Input: part model. Units: mm. Frame: model coordinates. Face numbers are marked on the shaded views. A direction names the side the tool comes from. Give positions to 0.01 mm unless a question says otherwise; leave off trailing zeros. Loops run counter-clockwise (first coordinate to the right, second up) from the corner with the lowest first, then second, coordinate; pieces in that order, holes last. Notation, with made-up numbers: (19.5, -20.5) - (38.5, -20.5) arc R19 cw to (38.5, -13.5) - close; hole circle Ø8 at (-40, -33). An arc over 180 degrees is marked (long way). Answer as a JSON object with one key per item and string values.
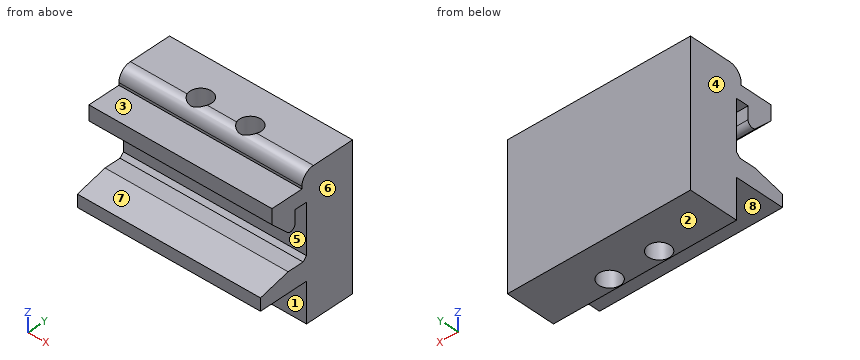
from build123d import *

# Parameters (mm, degrees)
BOSS_EXTRUDE1_DEPTH     = 37
SKETCH3_R               = 2.175
CUT_EXTRUDE1_DEPTH      = 9
CUT_EXTRUDE1_DEPTH_BACK = 21.75


with BuildPart() as part:
    # Sketch2 → Boss-Extrude1 (new body)
    with BuildSketch(Plane(origin=(0, 0, 0), x_dir=(0, 0, -1), z_dir=(1, 0, 0))):
        with BuildLine():
            Line((0, 0), (17.75, 0))
            Line((17.75, 0), (25.75, 0))
            Line((25.75, 0), (25.75, -10))
            Line((25.75, -10), (17.75, -10))
            Line((17.75, -10), (17.75, -20))
            Line((17.75, -20), (15.25, -20))
            Line((15.25, -20), (13.75, -14))
            Line((13.75, -14), (13.75, -10.75))
            Line((13.75, -10.75), (13, -10))
            Line((13, -10), (3, -10))
            Line((3, -10), (3, -12.5))
            Line((3, -12.5), (5.585786438, -12.5))
            ThreePointArc((5.585786438, -12.5), (6.50966597, -13.117316568), (6.292893219, -14.207106781))
            Line((6.292893219, -14.207106781), (3, -17.5))
            Line((3, -17.5), (0, -17.5))
            Line((0, -17.5), (0, -11))
            Line((0, -11), (-0.5, -11))
            ThreePointArc((-0.5, -11), (-2.267766953, -10.267766953), (-3, -8.5))
            Line((-3, -8.5), (-3, 0))
            Line((-3, 0), (0, 0))
        make_face()
    extrude(amount=BOSS_EXTRUDE1_DEPTH)

    # Sketch3 → Cut-Extrude1 (cut, two sides)
    with BuildSketch(Plane(origin=(0, 0, -17.75), x_dir=(-1, 0, 0), z_dir=(0, 0, -1))) as cut_extrude1_sk:
        with Locations((-23.5, -7.7)):
            Circle(SKETCH3_R)
        with Locations((-13.5, -7.7)):
            Circle(SKETCH3_R)
    extrude(amount=CUT_EXTRUDE1_DEPTH, mode=Mode.SUBTRACT)
    extrude(cut_extrude1_sk.sketch, amount=-CUT_EXTRUDE1_DEPTH_BACK, mode=Mode.SUBTRACT)


solid = part.part
Item 1: Material intervals for line 1 (X direction, y = -7.7, z = -12) (3 decimals); line 2 (Z direction, x = 26, y = -11.75); line 3 (X direction, y = -9.25, z = -15.25), sorted ascending. Write a range as [from, to].
Geometry check:
{"line 1": "x = [0, 11.325], [15.675, 21.325], [25.675, 37]", "line 2": "z = [-17.75, -13.75], [-3, 0]", "line 3": "x = [0, 11.97], [15.03, 21.97], [25.03, 37]"}
Item 2: Cut plane A-A (y = -7.7). Return loops of the section in (x, z) (3 decimals), then the cut area to 3 significant figures.
Geometry check:
{"outline": "(0, -25.75) - (11.325, -25.75) - (11.325, 3) - (0, 3) - close; (15.675, -25.75) - (21.325, -25.75) - (21.325, 3) - (15.675, 3) - close; (25.675, -25.75) - (37, -25.75) - (37, 3) - (25.675, 3) - close", "area": "814 mm2"}
Item 3: Access query for the marked faces 1, 2, 3, 4 and 5. Directions: +Z, -Z, +X, -X, +Y, -Y. A direction counts if a zero-diameter tool reaches every point of the face in a straight line with its end or side. Return the directions, or none.
Geometry check:
{"face 1": "-Z, +X, -X, -Y", "face 2": "-Z, +X, -X, +Y, -Y", "face 3": "+Z, +X, -X, -Y", "face 4": "+Z, -Z, -X, +Y, -Y", "face 5": "+X, -X"}
Item 4: Cut plane B-B (x = 23). Return loops of the section in (y, z), then the cut area to 3 significant figures.
Geometry check:
{"outline": "(-20, -17.75) - (-10, -17.75) - (-10, -25.75) - (-9.82, -25.75) - (-9.82, 2.63) arc R2.5 ccw to (-11, 0.5) - (-11, 0) - (-17.5, 0) - (-17.5, -3) - (-14.21, -6.29) arc R1 ccw to (-12.5, -5.59) - (-12.5, -3) - (-10, -3) - (-10, -13) - (-10.75, -13.75) - (-14, -13.75) - (-20, -15.25) - close; (-5.58, -25.75) - (0, -25.75) - (0, 3) - (-5.58, 3) - close", "area": "237 mm2"}
Item 5: Mould query, pull axis Z, two halves, no side actions, for the marked faces 6, 7 and 8. Classes: released by +Z, released by -Z, zero draft, split by the parting line, or undercut.
Geometry check:
{"face 6": "zero draft", "face 7": "undercut", "face 8": "released by -Z"}
Item 6: Cut plane D-D (x = 27.5). Return loops of the section in (y, z), then the cut area to 3 significant figures.
Geometry check:
{"outline": "(-20, -17.75) - (-10, -17.75) - (-10, -25.75) - (0, -25.75) - (0, 3) - (-8.5, 3) arc R2.5 ccw to (-11, 0.5) - (-11, 0) - (-17.5, 0) - (-17.5, -3) - (-14.21, -6.29) arc R1 ccw to (-12.5, -5.59) - (-12.5, -3) - (-10, -3) - (-10, -13) - (-10.75, -13.75) - (-14, -13.75) - (-20, -15.25) - close", "area": "359 mm2"}
Item 7: Contact query for flat-ended pins moving along their axis: P1, Ø1.6, axis at x = 18.5, y = -12.5, coming from the +Z side; P2, Ø2, axis at x = 15, y = -17.5, coming from the -Z side; P3, Ø2, axis at x = 28.5, z = -20, coming from the -Y side. Output: stop coordinate, or through.
Geometry check:
{"P1": "stops at z = 0", "P2": "stops at z = -17.75", "P3": "stops at y = -10"}
Item 8: Cut plane C-C (z = -21.5). Return loops of the section in (x, y) (3 decimals).
Geometry check:
{"outline": "(0, -10) - (37, -10) - (37, 0) - (0, 0) - close; hole circle Ø4.35 at (13.5, -7.7); hole circle Ø4.35 at (23.5, -7.7)"}
